from build123d import *

# Parameters (mm, degrees)
F0_W     = 230
F0_H     = 45
F1_DEPTH = 48
F3_DEPTH = 48
F5_DEPTH = 33
F6_R     = 4.5
F7_DEPTH = 15


with BuildPart() as f1:
    # F0 (on Top) → F1 (new body)
    with BuildSketch(Plane.XY):
        Rectangle(F0_W, F0_H)
    extrude(amount=F1_DEPTH)

    # F2 (on face) → F3 (cut, through all)
    with BuildSketch(Plane.XY.offset(48)):
        with BuildLine():
            ThreePointArc((-69.858372, 10.573861), (-88.148639, 15.512082), (-99.025, 0))
            ThreePointArc((-99.025, 0), (-88.148639, -15.512082), (-69.858372, -10.573861))
            ThreePointArc((-69.858372, -10.573861), (-66.02, -8.778061), (-62.181628, -10.573861))
            ThreePointArc((-62.181628, -10.573861), (-49.515, -16.5), (-36.848372, -10.573861))
            ThreePointArc((-36.848372, -10.573861), (-33.01, -8.778061), (-29.171628, -10.573861))
            ThreePointArc((-29.171628, -10.573861), (-16.505, -16.5), (-3.838372, -10.573861))
            ThreePointArc((-3.838372, -10.573861), (0, -8.778061), (3.838372, -10.573861))
            ThreePointArc((3.838372, -10.573861), (16.505, -16.5), (29.171628, -10.573861))
            ThreePointArc((29.171628, -10.573861), (33.01, -8.778061), (36.848372, -10.573861))
            ThreePointArc((36.848372, -10.573861), (49.515, -16.5), (62.181628, -10.573861))
            ThreePointArc((62.181628, -10.573861), (66.02, -8.778061), (69.858372, -10.573861))
            ThreePointArc((69.858372, -10.573861), (88.148639, -15.512082), (99.025, 0))
            ThreePointArc((99.025, 0), (88.148639, 15.512082), (69.858372, 10.573861))
            ThreePointArc((69.858372, 10.573861), (66.02, 8.778061), (62.181628, 10.573861))
            ThreePointArc((62.181628, 10.573861), (49.515, 16.5), (36.848372, 10.573861))
            ThreePointArc((36.848372, 10.573861), (33.01, 8.778061), (29.171628, 10.573861))
            ThreePointArc((29.171628, 10.573861), (16.505, 16.5), (3.838372, 10.573861))
            ThreePointArc((3.838372, 10.573861), (0, 8.778061), (-3.838372, 10.573861))
            ThreePointArc((-3.838372, 10.573861), (-16.505, 16.5), (-29.171628, 10.573861))
            ThreePointArc((-29.171628, 10.573861), (-33.01, 8.778061), (-36.848372, 10.573861))
            ThreePointArc((-36.848372, 10.573861), (-49.515, 16.5), (-62.181628, 10.573861))
            ThreePointArc((-62.181628, 10.573861), (-66.02, 8.778061), (-69.858372, 10.573861))
        make_face()
    extrude(amount=-F3_DEPTH, mode=Mode.SUBTRACT)

    # F4 (on face) → F5 (cut)
    with BuildSketch(Plane(origin=(0, 0, 0), x_dir=(1, 0, 0), z_dir=(0, 0, -1))):
        with BuildLine():
            Line((-115, -9.525), (-115, -9.472361))
            ThreePointArc((-115, -9.472361), (-115.499308, -9.511831), (-116, -9.525))
            Line((-116, -9.525), (-115, -9.525))
        make_face()
        with BuildLine():
            ThreePointArc((-115, -9.472361), (-106.475, 0), (-115, 9.472361))
            Line((-115, 9.472361), (-115, -9.472361))
        make_face()
        with BuildLine():
            Line((-115, 9.525), (-116, 9.525))
            ThreePointArc((-116, 9.525), (-115.499308, 9.511831), (-115, 9.472361))
            Line((-115, 9.472361), (-115, 9.525))
        make_face()
        with BuildLine():
            ThreePointArc((115, 9.472361), (115.499308, 9.511831), (116, 9.525))
            Line((116, 9.525), (115, 9.525))
            Line((115, 9.525), (115, 9.472361))
        make_face()
        with BuildLine():
            ThreePointArc((116, -9.525), (115.499308, -9.511831), (115, -9.472361))
            Line((115, -9.472361), (115, -9.525))
            Line((115, -9.525), (116, -9.525))
        make_face()
        with BuildLine():
            Line((115, -9.472361), (115, 9.472361))
            ThreePointArc((115, 9.472361), (106.475, 0), (115, -9.472361))
        make_face()
    extrude(amount=-F5_DEPTH, mode=Mode.SUBTRACT)

    # F6 (on face) → F7 (cut, through all)
    with BuildSketch(Plane(origin=(0, 0, 33), x_dir=(1, 0, 0), z_dir=(0, 0, -1))):
        with Locations((-116, 0)):
            Circle(F6_R)
        with Locations((116, 0)):
            Circle(F6_R)
    extrude(amount=-F7_DEPTH, mode=Mode.SUBTRACT)


solid = f1.part
Read the model definition and answer for the solid it produces. Units are mm, in the model's axes. A direction names the side the tool comes from. Coordinates: 2 decimals unless noted, no trailing zeros. Loops run counter-clockwise (first coordinate to the right, second up) from the corner with the lowest first, then second, coordinate; pieces in that order, holes last. Notation, with made-up numbers: (77.25, 61) -> (130.25, 61) arc R4 ccw to (130.25, 68) -> close; hole circle Ø5 at (-8, -24). An arc over 180 degrees is marked (long way). Answer in a Markdown table with one row per item.
Item 1: Straight lines are drawn through the part: line 1 along X through (y, z) = (-0.5, 28.5); line 2 along X through (y, z) = (-2, 43.5); line 3 along Y through (x, z) = (87.5, 17). For each, find the intervals that lie inside material, in ascending order. Write a range as [from, to].
Returned:
| item | result |
|---|---|
| line 1 | x = [-106.49, -99.02], [99.02, 106.49] |
| line 2 | x = [-111.97, -98.9], [98.9, 111.97] |
| line 3 | y = [-22.5, -15.73], [15.73, 22.5] |
Item 2: A cutting plane is placed at B-B on z = 37. Determine the outline of the cut face in (x, y) (3 decimals).
Returned:
| item | result |
|---|---|
| outline | (-115, -22.5) -> (115, -22.5) -> (115, -4.387) arc R4.5 cw to (115, 4.387) -> (115, 22.5) -> (-115, 22.5) -> (-115, 4.387) arc R4.5 cw to (-115, -4.387) -> close; hole (-69.858, -10.574) arc R5 cw to (-62.182, -10.574) arc R16.5 ccw to (-36.848, -10.574) arc R5 cw to (-29.172, -10.574) arc R16.5 ccw to (-3.838, -10.574) arc R5 cw to (3.838, -10.574) arc R16.5 ccw to (29.172, -10.574) arc R5 cw to (36.848, -10.574) arc R16.5 ccw to (62.182, -10.574) arc R5 cw to (69.858, -10.574) arc R16.5 ccw (long way) to (69.858, 10.574) arc R5 cw to (62.182, 10.574) arc R16.5 ccw to (36.848, 10.574) arc R5 cw to (29.172, 10.574) arc R16.5 ccw to (3.838, 10.574) arc R5 cw to (-3.838, 10.574) arc R16.5 ccw to (-29.172, 10.574) arc R5 cw to (-36.848, 10.574) arc R16.5 ccw to (-62.182, 10.574) arc R5 cw to (-69.858, 10.574) arc R16.5 ccw (long way) to start |
Item 3: A cutting plane is placed at A-A on x = -92. Determine the outline of the cut face in (y, z), plus the area to 3 significant figures.
Returned:
| item | result |
|---|---|
| outline | (-22.5, 0) -> (-13.51, 0) -> (-13.51, 48) -> (-22.5, 48) -> close; (13.51, 0) -> (22.5, 0) -> (22.5, 48) -> (13.51, 48) -> close |
| area | 863 mm^2 |
Item 4: This flat-tipped pin is pushed along its axis until it touches: P1, Ø7, axis at x = 112.5, y = 0, coming from the -Z side. Where does it stop, or does it pass through?
Returned:
| item | result |
|---|---|
| P1 | stops at z = 33 |
Item 5: A cutting plane is placed at C-C on x = 27. Determine the outline of the cut face in (y, z).
Returned:
| item | result |
|---|---|
| outline | (-22.5, 0) -> (-12.73, 0) -> (-12.73, 48) -> (-22.5, 48) -> close; (12.73, 0) -> (22.5, 0) -> (22.5, 48) -> (12.73, 48) -> close |
Item 6: For faces 1 (the flat face through (-115, -16, 24)), 2 (the cylindrical face through (32.95, -8.78, 24.34)), 3 (the flat face through (-111, 0, 33)), determine the directions among +Z, -Z, +X, -X, +Y, -Y from which every point of the face is accessible in a straight line to the end or side of a thin tool.
Returned:
| item | result |
|---|---|
| face 1 | +Z, -Z, -X, +Y, -Y |
| face 2 | +Z, -Z |
| face 3 | -Z, -X |
Item 7: A cutting plane is placed at D-D on z = 23.5. Determine the outline of the cut face in (x, y) (3 decimals).
Returned:
| item | result |
|---|---|
| outline | (-115, -22.5) -> (115, -22.5) -> (115, -9.472) arc R9.525 cw to (115, 9.472) -> (115, 22.5) -> (-115, 22.5) -> (-115, 9.472) arc R9.525 cw to (-115, -9.472) -> close; hole (-69.858, -10.574) arc R5 cw to (-62.182, -10.574) arc R16.5 ccw to (-36.848, -10.574) arc R5 cw to (-29.172, -10.574) arc R16.5 ccw to (-3.838, -10.574) arc R5 cw to (3.838, -10.574) arc R16.5 ccw to (29.172, -10.574) arc R5 cw to (36.848, -10.574) arc R16.5 ccw to (62.182, -10.574) arc R5 cw to (69.858, -10.574) arc R16.5 ccw (long way) to (69.858, 10.574) arc R5 cw to (62.182, 10.574) arc R16.5 ccw to (36.848, 10.574) arc R5 cw to (29.172, 10.574) arc R16.5 ccw to (3.838, 10.574) arc R5 cw to (-3.838, 10.574) arc R16.5 ccw to (-29.172, 10.574) arc R5 cw to (-36.848, 10.574) arc R16.5 ccw to (-62.182, 10.574) arc R5 cw to (-69.858, 10.574) arc R16.5 ccw (long way) to start |
Item 8: For a pull along X with two mould halves and no side action, classify faces 4 (the flat face through (111, 0, 33)), 5 (the cylindrical face through (-32.95, 8.78, 24.34)), 6 (the cylindrical face through (106.477, -0.195, 16.269)) as released by +X, released by -X, zero draft, split by the parting line, or undercut.
Returned:
| item | result |
|---|---|
| face 4 | zero draft |
| face 5 | undercut |
| face 6 | released by +X |
